Can you work these out from the model? Positions are in its coordinate system, mm. A direction names the side the tool comes from. Round coordinates to 2 decimals unless told otherwise and drop trailing zeros. Loops run counter-clockwise (first coordinate to the right, second up) from the corner with the lowest first, then second, coordinate; pieces in that order, holes last. Notation, with made-up numbers: M 46.25,11 L 74.25,11 A28 cw 74.25,49 Z; hole C -17,39 d2. An arc over 180 degrees is marked long. Return JSON: item names as keys, results as strings.
```python
from build123d import *

# Parameters (mm, degrees)
SKETCH2_R               = 6
BOSS_EXTRUDE1_DEPTH     = 14
SKETCH3_R               = 5
CUT_EXTRUDE1_DEPTH      = 4
SKETCH4_R               = 1.5
CUT_EXTRUDE2_DEPTH      = 7
CUT_EXTRUDE2_DEPTH_BACK = 7
SKETCH7_W               = 8
SKETCH7_H               = 9
CUT_EXTRUDE5_DEPTH      = 7.0000001
CUT_EXTRUDE5_DEPTH_BACK = 7.0000001
SKETCH8_R               = 1.5
CUT_EXTRUDE6_DEPTH      = 7.0000001
CUT_EXTRUDE6_DEPTH_BACK = 7.0000001


with BuildPart() as part:
    # Sketch2 → Boss-Extrude1 (new body)
    with BuildSketch(Plane.XY):
        Circle(SKETCH2_R)
    extrude(amount=BOSS_EXTRUDE1_DEPTH)

    # Sketch3 → Cut-Extrude1 (cut)
    with BuildSketch(Plane.XY.offset(14)):
        Circle(SKETCH3_R)
    extrude(amount=-CUT_EXTRUDE1_DEPTH, mode=Mode.SUBTRACT)

    # Sketch4 → Cut-Extrude2 (cut, two sides)
    with BuildSketch(Plane(origin=(0, 0, 0), x_dir=(0, 0, -1), z_dir=(1, 0, 0))) as cut_extrude2_sk:
        with Locations((-12, 0)):
            Circle(SKETCH4_R)
    extrude(amount=CUT_EXTRUDE2_DEPTH, mode=Mode.SUBTRACT)
    extrude(cut_extrude2_sk.sketch, amount=-CUT_EXTRUDE2_DEPTH_BACK, mode=Mode.SUBTRACT)

    # Sketch7 → Cut-Extrude5 (cut, two sides)
    with BuildSketch(Plane(origin=(0, 0, 0), x_dir=(1, 0, 0), z_dir=(0, 1, 0))) as cut_extrude5_sk:
        with Locations((0.10757358, -5.111243205)):
            Rectangle(SKETCH7_W, SKETCH7_H)
    extrude(amount=CUT_EXTRUDE5_DEPTH, mode=Mode.SUBTRACT)
    extrude(cut_extrude5_sk.sketch, amount=-CUT_EXTRUDE5_DEPTH_BACK, mode=Mode.SUBTRACT)

    # Sketch8 → Cut-Extrude6 (cut, two sides)
    with BuildSketch(Plane(origin=(0, 0, 0), x_dir=(0, 0, -1), z_dir=(1, 0, 0))) as cut_extrude6_sk:
        with Locations((-5.111243205, 0)):
            Circle(SKETCH8_R)
    extrude(amount=CUT_EXTRUDE6_DEPTH, mode=Mode.SUBTRACT)
    extrude(cut_extrude6_sk.sketch, amount=-CUT_EXTRUDE6_DEPTH_BACK, mode=Mode.SUBTRACT)


solid = part.part
```
Q1. Suppose I cut it at D-D, the plane x = -4.5. Please give me the cut outline in (y, z), plus the area to 3 significant figures.
Results:
{"outline": "M -3.97,0 L 3.97,0 L 3.97,14 L 2.18,14 L 2.18,10 L -2.18,10 L -2.18,14 L -3.97,14 Z; hole C 0,5.11 d3", "area": "86.6 mm2"}
Q2. Suppose I cut it at B-B, the plane x = 0. Please give me the cut outline in (y, z), plus the area to 3 significant figures.
Results:
{"outline": "M -6,0 L 6,0 L 6,0.61 L -6,0.61 Z; M -6,9.61 L 6,9.61 L 6,14 L 5,14 L 5,10 L -5,10 L -5,14 L -6,14 Z", "area": "20.0 mm2"}
Q3. Suppose I cut it at A-A, the plane y = 0. Please give me the cut outline in (x, z).
Results:
{"outline": "M -6,0 L 6,0 L 6,3.61 L 4.11,3.61 L 4.11,0.61 L -3.89,0.61 L -3.89,3.61 L -6,3.61 Z; M -6,6.61 L -3.89,6.61 L -3.89,9.61 L 4.11,9.61 L 4.11,6.61 L 6,6.61 L 6,10.5 L 5,10.5 L 5,10 L -5,10 L -5,10.5 L -6,10.5 Z; M -6,13.5 L -5,13.5 L -5,14 L -6,14 Z; M 5,13.5 L 6,13.5 L 6,14 L 5,14 Z"}
Q4. If I drill on line 1 along Z through (x, y) = (-0.5, 3); line 2 along X through (y, z) = (0.25, 1.5); line 3 along X through (y, z) = (1.75, 13), over which ranges is the centre line in solid material (lowest first)?
Results:
{"line 1": "z = 0 to 0.61, 9.61 to 10", "line 2": "x = -5.99 to -3.89, 4.11 to 5.99", "line 3": "x = -5.74 to -4.68, 4.68 to 5.74"}
Q5. I'm going to push flat-ended pins straight in: pin 1 Ø4 at (x, y) = (-1.5, 2.5) entering from +Z; pin 2 Ø1.8 at (y, z) = (0, 12) entering from -X; pin 3 Ø4 at (y, z) = (-2, 4.5) entering from -X; pin 4 Ø4 at (y, z) = (4.5, 5) entering from -X. Where does each tip first touch, or does it pass through?
Results:
{"pin 1": "stops at z = 10", "pin 2": "passes through", "pin 3": "stops at x = -6", "pin 4": "stops at x = -5.45"}
Q6. Suppose I cut it at C-C, the plane z = 10.75. Please give me the cut outline in (x, y), plus the area to 3 significant figures.
Results:
{"outline": "M -5.94,-0.83 A6 ccw 5.94,-0.83 L 4.93,-0.83 A5 cw -4.93,-0.83 Z; M -5.94,0.83 L -4.93,0.83 A5 cw 4.93,0.83 L 5.94,0.83 A6 ccw Z", "area": "31.2 mm2"}
Q7. Thinking about a two-plate mould opening in Z: for faces 4 (the flat face through (-3.892, 0, 7)), 5 (the flat face through (0, 0, 0)), 6 (the flat face through (-4, 4, 14)), which applies, pulls with the +Z half, pulls with the -Z half, needs draft (parallel to the pull), parting line crosses it, or undercut?
Results:
{"face 4": "undercut", "face 5": "pulls with the -Z half", "face 6": "pulls with the +Z half"}
Q8. On a 3-axis mill with a long thin cutter (end or side, diameter ignored), from which of +Z, -Z, +X, -X, +Y, -Y can I reach the whole of each face in a straight line? I mean faces 1 (the cylindrical face through (5.04, 0.07, 6.61)), 2 (the flat face through (0, 0, 10)), 3 (the flat face through (0, 0, 0.611)). Say none if no direction works.
Results:
{"face 1": "+X, -X", "face 2": "+Z", "face 3": "+Y, -Y"}
